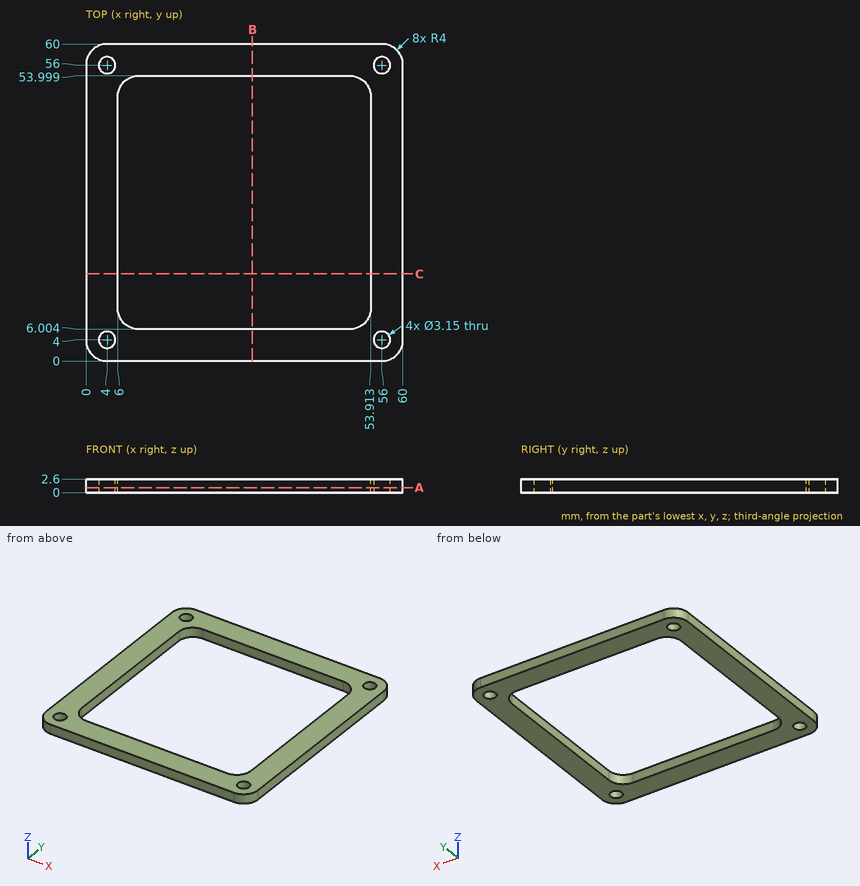
Study the drawing (mm; zero at the part's minimum x, y, z) and answer. Round coordinates to 2 decimals unless told otherwise and drop trailing zeros. Order: outer loops, then holes, each group sorted by start corner. A loop starts at its lowest first (then second) coordinate and runs counter-clockwise, first axis right, second up. Notation, with made-up numbers: (61, 44) -> (120, 44) arc R32 ccw to (120, 83) -> close; hole circle Ø7 at (28.25, -2). An arc over 180 degrees is marked (long way). Answer as CSV lines item,"result". Start each with the question number.
(1) The part is cut by section B-B (x = 31.5). Determine the outline of the cut face in (y, z), then the cut area to 3 significant figures.
(2) Find the intervals of material crossed by probe 1 along Y at (x, z) = (4, 0.8) (1 decimal); probe 2 along X at (y, z) = (37, 0.35); probe 3 along Y at (x, z) = (44.5, 2.2), in increasing order. Write a range as from..to.
(3) The part is cut by section C-C (y = 16.5). Determine the outline of the cut face in (x, z).
(4) Flat-ended cylindrical pins translate along their axes: pin 1 Ø2.5 at (x, y) = (4, 56) entering from -Z; pin 2 Ø3.5 at (x, y) = (4, 4) entering from +Z. Find the tip coordinate at first contact, or state that the pin passes through.
(5) The part is cut by section A-A (z = 0.95). Count the separate pieces of the cut face and the enclosed holes in it, then the cut area to 3 significant figures.
Evaluation:
1,outline,"(0, 0) -> (6, 0) -> (6, 2.6) -> (0, 2.6) -> close; (54, 0) -> (60, 0) -> (60, 2.6) -> (54, 2.6) -> close"
1,area,"31.2 mm²"
2,probe 1,"0..2.4, 5.6..54.4, 57.6..60"
2,probe 2,"0..6, 53.91..60"
2,probe 3,"0..6, 54..60"
3,outline,"(0, 0) -> (6, 0) -> (6, 2.6) -> (0, 2.6) -> close; (53.91, 0) -> (60, 0) -> (60, 2.6) -> (53.91, 2.6) -> close"
4,pin 1,"through"
4,pin 2,"z = 2.6"
5,separate pieces,"1"
5,enclosed holes,"5"
5,area,"1,270 mm²"
